Can you work these out from the drawing? Everything is in mm from the part's minimum corner. Round coordinates to 2 decimals unless told otherwise and drop trailing zeros. Loops run counter-clockwise (first coordinate to the right, second up) from the corner with the lowest first, then second, coordinate; pieces in that order, holes last. Notation, with made-up numbers: M -35.75,-40 L -4.75,-40 A8 cw -4.75,-27 Z; hole C 62.25,-36.5 d11. An arc over 180 degrees is marked long. Answer in a Markdown table with one row per item.
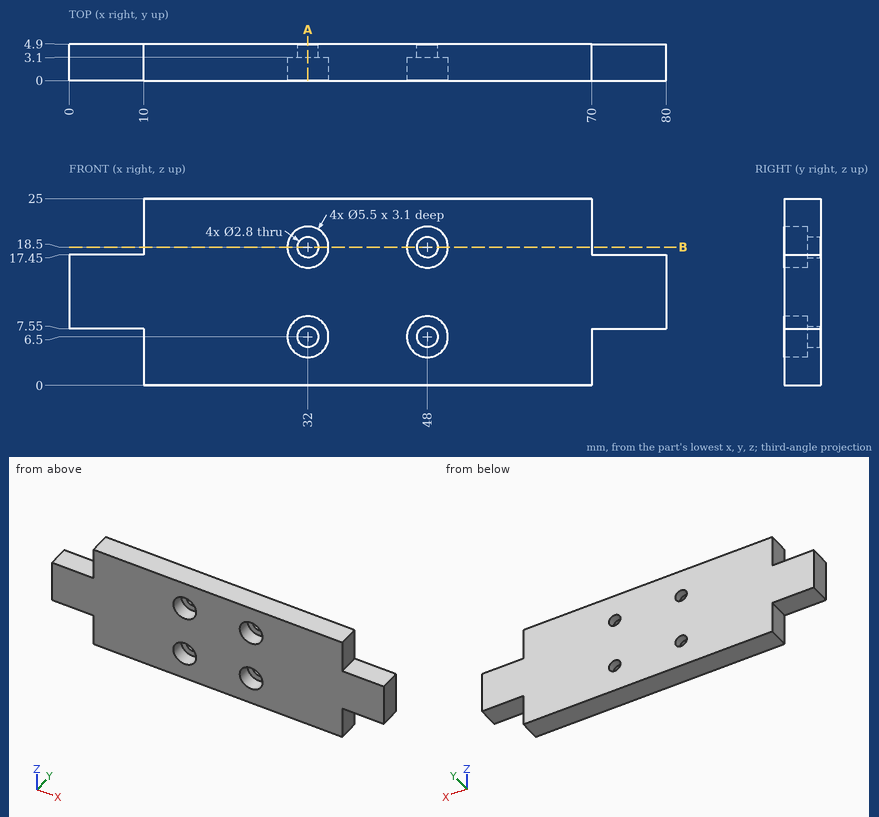
1) I need wall thicknesses on line 1 (X direction, y = 3.65, z = 18.5); line 2 (Z direction, x = 32, y = 4.3); line 3 (X direction, y = 1.8, z = 21). Which ranges of each line are inside material? Lowest first, please.
Computed:
| item | result |
|---|---|
| line 1 | x = 10 to 30.6, 33.4 to 46.6, 49.4 to 70 |
| line 2 | z = 0 to 5.1, 7.9 to 17.1, 19.9 to 25 |
| line 3 | x = 10 to 30.85, 33.15 to 46.85, 49.15 to 70 |
2) Will these pins go through, and if not, where does the flat tip stop? P1, Ø1.6, axis at x = 32, z = 7.5, coming from the -Y side; P2, Ø7, axis at x = 48, z = 6.5, coming from the +Y side; P3, Ø2.5, axis at x = 6.5, y = 1.5, coming from the +Z side; P4, Ø2.5, axis at y = 3.5, z = 20.5, coming from the -X side.
Computed:
| item | result |
|---|---|
| P1 | stops at y = 3.1 |
| P2 | stops at y = 4.9 |
| P3 | stops at z = 17.45 |
| P4 | stops at x = 10 |
3) I want a section at B-B, the plane z = 18.5. Please give me the cut outline in (x, y), plus the area to 3 significant figures.
Computed:
| item | result |
|---|---|
| outline | M 10,0 L 29.25,0 L 29.25,3.1 L 30.6,3.1 L 30.6,4.9 L 10,4.9 Z; M 33.4,3.1 L 34.75,3.1 L 34.75,0 L 45.25,0 L 45.25,3.1 L 46.6,3.1 L 46.6,4.9 L 33.4,4.9 Z; M 49.4,3.1 L 50.75,3.1 L 50.75,0 L 70,0 L 70,4.9 L 49.4,4.9 Z |
| area | 250 mm² |
4) I want a section at A-A, the plane x = 32. Please give me the cut outline in (y, z).
Computed:
| item | result |
|---|---|
| outline | M 0,0 L 4.9,0 L 4.9,5.1 L 3.1,5.1 L 3.1,3.75 L 0,3.75 Z; M 0,9.25 L 3.1,9.25 L 3.1,7.9 L 4.9,7.9 L 4.9,17.1 L 3.1,17.1 L 3.1,15.75 L 0,15.75 Z; M 0,21.25 L 3.1,21.25 L 3.1,19.9 L 4.9,19.9 L 4.9,25 L 0,25 Z |
